```python
from build123d import *

# Parameters (mm, degrees)
SKETCH2_R           = 2.15
BOSS_EXTRUDE2_DEPTH = 5
SKETCH2_4_R         = 2.5
BOSS_EXTRUDE3_DEPTH = 10
SKETCH2_5_R         = 2.15
CUT_EXTRUDE1_DEPTH  = 10


with BuildPart() as part:
    # Sketch2 → Boss-Extrude2 (new body)
    with BuildSketch(Plane(origin=(0, 0, 0), x_dir=(1, 0, 0), z_dir=(0, 1, 0))):
        with BuildLine():
            ThreePointArc((41.396346652, -14.911153002), (88.805627965, 0), (41.396346652, 14.911153002))
            add(Edge.make_bspline(
                [(41.396346652, 14.911153002), (35.610115035, 8.935267229), (30.816373967, 8.824209594), (28.225205258, 7.191755049)],
                knots=[0.924562573, 0.924562573, 0.924562573, 0.924562573, 1.924562573, 1.924562573, 1.924562573, 1.924562573], degree=3))
            ThreePointArc((28.225205258, 7.191755049), (24.256061614, 0), (28.225205258, -7.191755049))
            add(Edge.make_bspline(
                [(28.225205258, -7.191755049), (30.816373967, -8.824209594), (35.610115035, -8.935267229), (41.396346652, -14.911153002)],
                knots=[0, 0, 0, 0, 1, 1, 1, 1], degree=3))
        make_face()
        with Locations(Location((83.805627965, 0, 0), (0, 0, 270))):
            Circle(SKETCH2_R, mode=Mode.SUBTRACT)
    extrude(amount=BOSS_EXTRUDE2_DEPTH)

    # Sketch2<4> → Boss-Extrude3 (add)
    with BuildSketch(Plane(origin=(0, 0, 0), x_dir=(1, 0, 0), z_dir=(0, 1, 0))):
        with Locations(Location((32.756061614, 0, 0), (0, 0, 270))):
            Circle(SKETCH2_4_R)
        with BuildLine():
            ThreePointArc((41.396346652, 14.911153002), (88.805627965, 0), (41.396346652, -14.911153002))
            ThreePointArc((41.396346652, -14.911153002), (44, 0), (41.396346652, 14.911153002))
        make_face()
    extrude(amount=BOSS_EXTRUDE3_DEPTH)

    # Sketch2<5> → Cut-Extrude1 (cut)
    with BuildSketch(Plane(origin=(0, 0, 0), x_dir=(1, 0, 0), z_dir=(0, 1, 0))):
        with Locations(Location((83.805627965, 0, 0), (0, 0, 90))):
            Circle(SKETCH2_5_R)
    extrude(amount=CUT_EXTRUDE1_DEPTH, mode=Mode.SUBTRACT)


solid = part.part
```
Verification items for the finished model (mm, model axes). A direction names the side the tool comes from. Round coordinates to 2 decimals unless told otherwise and drop trailing zeros. Write each loop counter-clockwise with the first axis right and the second up, starting at its lowest first coordinate (ties: lowest second). Pieces come first, ordered by that corner, then holes. Notation, with made-up numbers: (-16, -25.75) - (36, -25.75) arc R16 ccw to (36, -10.75) - close; hole circle Ø9 at (86.25, -13.5). An arc over 180 degrees is marked (long way). Answer as a JSON object with one key per item and string values. Group by question number.
Q1. Section check A-A, the plane z = 0. Enter the section's corners in (x, y).
Q2. Section check C-C, the plane x = 47. Enter the section's corners in (y, z), plus the area to 3 significant figures.
Q3. Mould release check, pull along X, two halves, no side actions. Record for faces 1 (the cylindrical face through (85.713, 4.93, -0.992)), 2 (the cylindrical face through (24.257, 2.465, -0.12)), 3 (the flat face through (57, 0, 0)): released by +X, released by -X, zero draft, split by the parting line, or undercut.
Q4. Go/stop test with flat-tipped pins: pin 1 Ø4 at (x, z) = (83.81, 0) entering from -Y; pin 2 Ø1 at (y, z) = (7, -4.5) entering from +X; pin 3 Ø4 at (x, y) = (47.5, 1.5) entering from -Z; pin 4 Ø1.5 at (x, y) = (56.5, 6) entering from -Z. Record where each tip stops, or that it passes through.
Q5. Tool access check on faces 4 (the flat face through (33, 10, 0)), 5 (the cylindrical face through (30.316, 7.465, -0.542)). Record the directions out of +Z, -Z, +X, -X, +Y, -Y that give a thin tool (end or side, any length) a straight path to the whole face; none if there is none.
Q6. Section check D-D, the plane x = 57. Enter the section's corners in (y, z), plus the area to 3 significant figures.
Q7. Thickness scan on line 1 (X direction, y = 3.5, z = 1.5); line 2 (Z direction, x = 63, y = 8.5); line 3 (Y direction, x = 32, z = -7.5). Record the ranges inside material, lowest first.
Q8. Section check B-B, the plane y = 7.5. Enter the section's corners in (x, z).
Found:
{
 "1": {"outline": "(24.26, 0) - (81.66, 0) - (81.66, 10) - (44, 10) - (44, 5) - (35.26, 5) - (35.26, 10) - (30.26, 10) - (30.26, 5) - (24.26, 5) - close; (85.96, 0) - (88.81, 0) - (88.81, 10) - (85.96, 10) - close"},
 "2": {"outline": "(0, -20.74) - (10, -20.74) - (10, 20.74) - (0, 20.74) - close", "area": "415 mm^2"},
 "3": {"face 1": "undercut", "face 2": "released by -X", "face 3": "zero draft"},
 "4": {"pin 1": "passes through", "pin 2": "stops at x = 88.5", "pin 3": "stops at z = -22.42", "pin 4": "stops at z = -25.46"},
 "5": {"face 4": "+Z, -Z, +X, -X, +Y", "face 5": "+Y"},
 "6": {"outline": "(0, -25.41) - (10, -25.41) - (10, 25.41) - (0, 25.41) - close", "area": "508 mm^2"},
 "7": {"line 1": "x = 24.39 to 82.27, 85.35 to 88.76", "line 2": "z = -26.05 to 26.05", "line 3": "y = 0 to 5"},
 "8": {"outline": "circle Ø5 at (32.76, 0); (41.4, -14.91) arc R26.05 ccw (long way) to (41.4, 14.91) arc R44 cw to start; hole circle Ø4.3 at (83.81, 0)"}
}
